from build123d import *

# Parameters (mm, degrees)
F0_W     = 120
F0_H     = 35
F0_R     = 10
F1_DEPTH = 10
F2_R     = 5
F3_R     = 10
F4_DEPTH = 25


with BuildPart() as f1:
    # F0 (on Top) → F1 (new body)
    with BuildSketch(Plane.XY):
        Rectangle(F0_W, F0_H)
        with Locations((-45, 0)):
            Circle(F0_R, mode=Mode.SUBTRACT)
    extrude(amount=F1_DEPTH)

    # F2
    f2_edges = [f1.edges().sort_by_distance(p)[0] for p in [
        (-60, -17.5, 5),
        (60, -17.5, 5),
        (60, 17.5, 5),
        (-60, 17.5, 5),
    ]]
    fillet(f2_edges, radius=F2_R)

    # F3 (on face) → F4 (join)
    with BuildSketch(Plane.XY.offset(10)):
        with BuildLine():
            ThreePointArc((55, -17.5), (58.535534, -16.035534), (60, -12.5))
            Line((60, -12.5), (60, 12.5))
            ThreePointArc((60, 12.5), (58.535534, 16.035534), (55, 17.5))
            Line((55, 17.5), (-55, 17.5))
            ThreePointArc((-55, 17.5), (-58.535534, 16.035534), (-60, 12.5))
            Line((-60, 12.5), (-60, -12.5))
            ThreePointArc((-60, -12.5), (-58.535534, -16.035534), (-55, -17.5))
            Line((-55, -17.5), (55, -17.5))
        make_face()
        with Locations((-45, 0)):
            Circle(F3_R, mode=Mode.SUBTRACT)
    extrude(amount=F4_DEPTH)


solid = f1.part
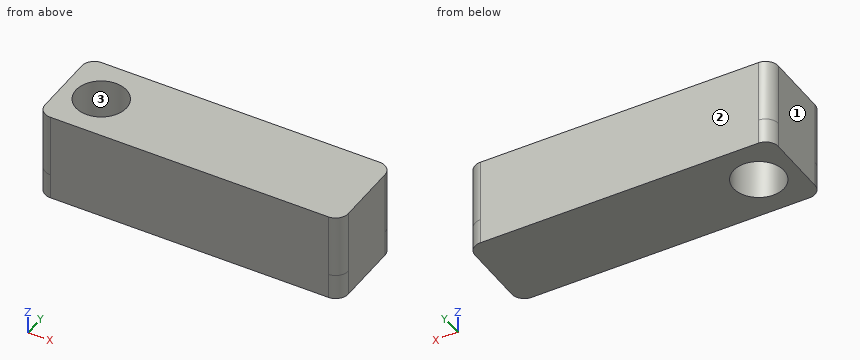
Can you work these out from the model? Positions are in its coordinate system, mm. Face numbers are marked on the shaded views. Give positions to 0.01 mm unless a question says otherwise; leave off trailing zeros. Order: outer loops, then holes, each group sorted by start corner. A loop starts at its lowest first (then second) coordinate and runs counter-clockwise, first axis right, second up. Notation, with made-up numbers: M -16,-31.5 L 23,-31.5 A18 cw 23,2.5 Z; hole C -10,-36.5 d9. An arc over 180 degrees is marked long. Use a Markdown table: item, result. Add a question column.
Item 1: Suppose I cut it at A-A (x = -45). List the corners of the cut face in (y, z) for me.
Item 2: Suppose I cut it at B-B (z = 18). List the corners of the cut face in (x, y) for me.
Item 3: Suppose I cut it at C-C (y = 0). List the corners of the cut face in (x, z) for me.
Item 4: We'd pull the mould along X, two halves only. Please class the marked faces 1, 2 and 3: +X half, -X half, draft (parallel to the pull), parting line (faces both ways), or undercut.
Item 5: If I drill on L1, parallel to Y at x = -45, z = 18; L2, parallel to X at y = 6, z = 28; L3, parallel to X at y = -5.5, z = 24, over which ranges is the centre line in solid material (lowest first)? Write a range as [from, to].
Answer sheet:
| question | item | result |
|---|---|---|
| 1 | outline | M -17.5,0 L -10,0 L -10,35 L -17.5,35 Z; M 10,0 L 17.5,0 L 17.5,35 L 10,35 Z |
| 2 | outline | M -60,-12.5 A5 ccw -55,-17.5 L 55,-17.5 A5 ccw 60,-12.5 L 60,12.5 A5 ccw 55,17.5 L -55,17.5 A5 ccw -60,12.5 Z; hole C -45,0 d20 |
| 3 | outline | M -60,0 L -55,0 L -55,35 L -60,35 Z; M -35,0 L 60,0 L 60,35 L -35,35 Z |
| 4 | face 1 | -X half |
| 4 | face 2 | draft |
| 4 | face 3 | undercut |
| 5 | L1 | y = [-17.5, -10], [10, 17.5] |
| 5 | L2 | x = [-60, -53], [-37, 60] |
| 5 | L3 | x = [-60, -53.35], [-36.65, 60] |
